```python
from build123d import *

# Parameters (mm, degrees)
SKETCH_1_R          = 10
SKETCH_1_R_2        = 8
EXTRUDE_1_DEPTH     = 10
EXTRUDE_2_DEPTH     = 6
SKETCH_3_R          = 14
CUT_EXTRUDE_1_DEPTH = 4
FILLET_1_R          = 2


with BuildPart() as part:
    # Эскиз1 → Бобышка-Вытянуть1 (new body)
    with BuildSketch(Plane.XY):
        Circle(SKETCH_1_R)
        Circle(SKETCH_1_R_2, mode=Mode.SUBTRACT)
    extrude(amount=EXTRUDE_1_DEPTH)

    # Эскиз2 → Бобышка-Вытянуть2 (add)
    with BuildSketch(Plane.XY.offset(10)):
        with BuildLine():
            ThreePointArc((3.876767447, 16.985227976), (0, 20), (-3.876767447, 16.985227976))
            ThreePointArc((-3.876767447, 16.985227976), (-8.677674782, 18.019377358), (-10.862461002, 13.621095265))
            ThreePointArc((-10.862461002, 13.621095265), (-15.636629649, 12.469796037), (-15.696710936, 7.559137585))
            ThreePointArc((-15.696710936, 7.559137585), (-19.498558244, 4.450418679), (-17.422034762, 0))
            ThreePointArc((-17.422034762, 0), (-19.498558244, -4.450418679), (-15.696710936, -7.559137585))
            ThreePointArc((-15.696710936, -7.559137585), (-15.636629649, -12.469796037), (-10.862461002, -13.621095265))
            ThreePointArc((-10.862461002, -13.621095265), (-8.677674782, -18.019377358), (-3.876767447, -16.985227976))
            ThreePointArc((-3.876767447, -16.985227976), (0, -20), (3.876767447, -16.985227976))
            ThreePointArc((3.876767447, -16.985227976), (8.677674782, -18.019377358), (10.862461002, -13.621095265))
            ThreePointArc((10.862461002, -13.621095265), (15.636629649, -12.469796037), (15.696710936, -7.559137585))
            ThreePointArc((15.696710936, -7.559137585), (19.498558244, -4.450418679), (17.422034762, 0))
            ThreePointArc((17.422034762, 0), (19.498558244, 4.450418679), (15.696710936, 7.559137585))
            ThreePointArc((15.696710936, 7.559137585), (15.636629649, 12.469796037), (10.862461002, 13.621095265))
            ThreePointArc((10.862461002, 13.621095265), (8.677674782, 18.019377358), (3.876767447, 16.985227976))
        make_face()
    extrude(amount=EXTRUDE_2_DEPTH)

    # Эскиз3 → Вырез-Вытянуть1 (cut)
    with BuildSketch(Plane.XY.offset(16)):
        Circle(SKETCH_3_R)
    extrude(amount=-CUT_EXTRUDE_1_DEPTH, mode=Mode.SUBTRACT)

    # Скругление1
    fillet_1_edges = [part.edges().sort_by_distance(p)[0] for p in [
        (-14, 0, 12),
    ]]
    fillet(fillet_1_edges, radius=FILLET_1_R)


solid = part.part
```
Part model, mm, in its own coordinate system. A direction names the side the tool comes from. Round coordinates to 2 decimals unless told otherwise and drop trailing zeros. Write each loop counter-clockwise with the first axis right and the second up, starting at its lowest first coordinate (ties: lowest second). Pieces come first, ordered by that corner, then holes.
Item 1: Drop flat-ended pins along their axis: pin 1 Ø2 at (y, z) = (0.5, 2) entering from +X; pin 2 Ø1 at (x, y) = (2, 11) entering from -Z; pin 3 Ø3 at (x, z) = (-6.5, 11) entering from +Y. Give the stop position or say it passes through.
Results:
pin 1: stops at x = 10
pin 2: stops at z = 10
pin 3: stops at y = 18.42
Item 2: Two-plate mould, pull along X, no slides. Class faces 4 (the flat face through (0, 8.2, 0)), 5 (the cylindrical face through (-8.74, -17.99, 12.96)), 6 (the cylindrical face through (-2.17, -9.76, 4.93)), 7 (the flat face through (0, 0, 10)): +X half, -X half, draft (parallel to the pull), parting line (faces both ways), or undercut.
Results:
face 4: draft
face 5: undercut
face 6: parting line
face 7: undercut
Item 3: Cut at B-B, the plane y = 17.5. Give the cut face in (x, z).
Results:
outline: (-9.49, 10) - (-4.4, 10) - (-4.4, 16) - (-9.49, 16) - close; (-3.71, 10) - (3.71, 10) - (3.71, 16) - (-3.71, 16) - close; (4.4, 10) - (9.49, 10) - (9.49, 16) - (4.4, 16) - close
Item 4: Cut at D-D, the plane z = 10.5. Give the cut face in (x, y), plus the area to 3 significant figures.
Results:
outline: (-17.42, 0) arc R4 ccw to (-15.7, -7.56) arc R4 ccw to (-10.86, -13.62) arc R4 ccw to (-3.88, -16.99) arc R4 ccw to (3.88, -16.99) arc R4 ccw to (10.86, -13.62) arc R4 ccw to (15.7, -7.56) arc R4 ccw to (17.42, 0) arc R4 ccw to (15.7, 7.56) arc R4 ccw to (10.86, 13.62) arc R4 ccw to (3.88, 16.99) arc R4 ccw to (-3.88, 16.99) arc R4 ccw to (-10.86, 13.62) arc R4 ccw to (-15.7, 7.56) arc R4 ccw to start
area: 1,160 mm2
Item 5: Probe L1, parallel to Y at x = 0, z = 4; L2, parallel to Z at x = 6.5, y = -10; L3, parallel to Z at x = -11.5, y = 13.5. List the from-to ranges inside material, lowest first.
Results:
L1: y = -10 to -8, 8 to 10
L2: z = 10 to 12
L3: z = 10 to 16
Item 6: Which spindle directions (+Z, -Z, +X, -X, +Y, -Y) get a long thin tool onto all of the face, cutting with end or side? Do faces 1 (the flat face through (13, -6, 16)), 2 (the cylindrical face through (12.932, -5.362, 15.014)), 3 (the cylindrical face through (-1.73, -7.81, 4.93)). Say none if no direction does.
Results:
face 1: +Z, +X, -X, +Y, -Y
face 2: +Z
face 3: -Z
Item 7: Cut at A-A, the plane x = 0. Give the cut face in (y, z).
Results:
outline: (-20, 10) - (-10, 10) - (-10, 0) - (-8, 0) - (-8, 10) - (8, 10) - (8, 0) - (10, 0) - (10, 10) - (20, 10) - (20, 16) - (14, 16) - (14, 14) arc R2 cw to (12, 12) - (-12, 12) arc R2 cw to (-14, 14) - (-14, 16) - (-20, 16) - close
Item 8: Cut at C-C, the plane z = 13. Give the cut face in (x, y).
Results:
outline: (-17.42, 0) arc R4 ccw to (-15.7, -7.56) arc R4 ccw to (-10.86, -13.62) arc R4 ccw to (-3.88, -16.99) arc R4 ccw to (3.88, -16.99) arc R4 ccw to (10.86, -13.62) arc R4 ccw to (15.7, -7.56) arc R4 ccw to (17.42, 0) arc R4 ccw to (15.7, 7.56) arc R4 ccw to (10.86, 13.62) arc R4 ccw to (3.88, 16.99) arc R4 ccw to (-3.88, 16.99) arc R4 ccw to (-10.86, 13.62) arc R4 ccw to (-15.7, 7.56) arc R4 ccw to start; hole circle Ø27.46 at (0, 0)
